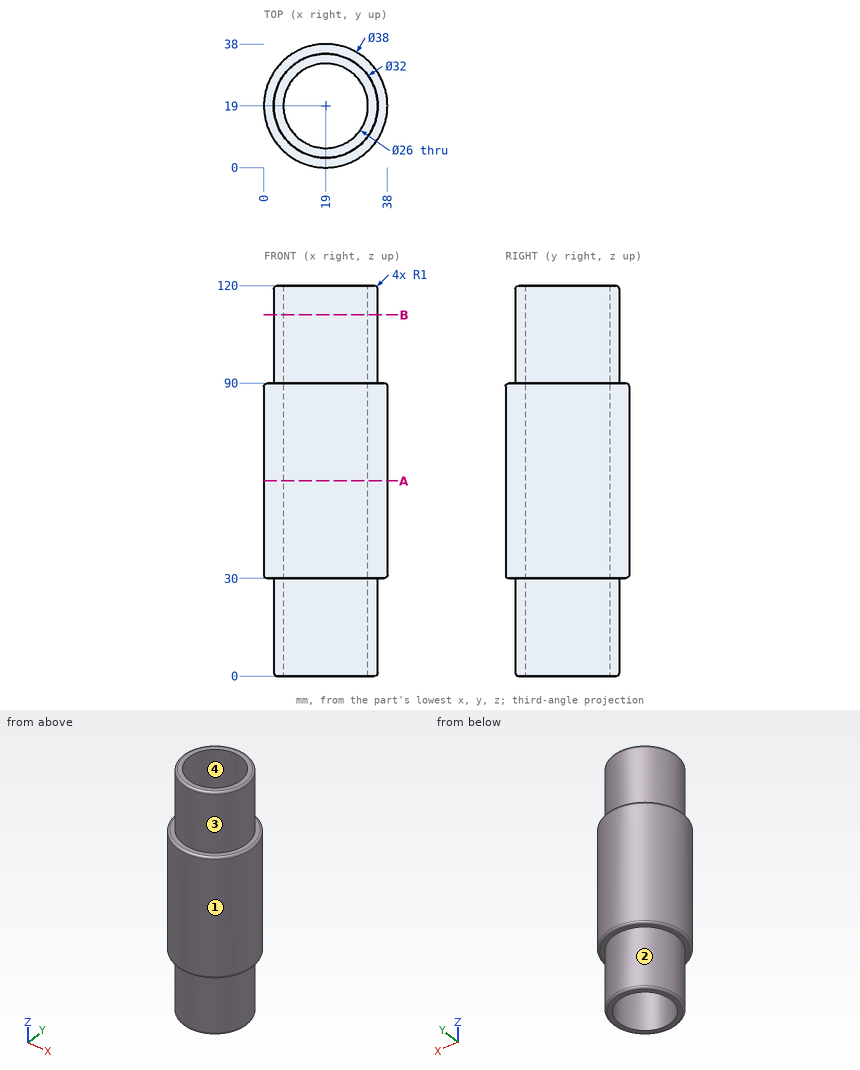
Can you work these out from the drawing? Everything is in mm from the part's minimum corner. A direction names the side the tool comes from. Round coordinates to 2 decimals unless told otherwise and drop trailing zeros. Loops run counter-clockwise (first coordinate to the right, second up) from the corner with the lowest first, then second, coordinate; pieces in that order, holes last. Notation, with made-up numbers: (78.25, 67) - (125.25, 67) arc R15 ccw to (125.25, 79) - close; hole circle Ø4 at (44.5, 52). An arc over 180 degrees is marked (long way). One line per question, with ' | ' between items. Start each with the question number.
Q1. Will these pins go through, and if not, where does the flat tip stop? pin 1 (4 mm diameter, centred on x = 20.5, z = 88.5, fed in from -Y); pin 2 (8 mm diameter, centred on x = 9, z = 54.5, fed in from -Y); pin 3 (8 mm diameter, centred on y = 29, z = 71, fed in from -X).
Q2. I want a section at B-B (z = 111). Write out the boundary of the cut face in (x, y).
Q3. We'd pull the mould along Y, two halves only. Please class the marked faces 3 and 4: +Y half, -Y half, draft (parallel to the pull), parting line (faces both ways), or undercut.
Q4. I want a section at A-A (z = 60). Write out the boundary of the cut face in (x, y).
Q5. Please list where these lines run through material, in increasing order: line 1 (Y direction, x = 19, z = 92.5); line 2 (Y direction, x = 19, z = 74.5); line 3 (X direction, y = 7, z = 72.5). Write a range as [from, to].
Q6. For the marked faces 1 and 2, which set-ups out of +Z, -Z, +X, -X, +Y, -Y let a thin tool reach every point of the face, with its end or its side?
Response values:
1) pin 1: stops at y = 0 | pin 2: stops at y = 0.97 | pin 3: stops at x = 0.97
2) outline: circle Ø32 at (19, 19); hole circle Ø26 at (19, 19)
3) face 3: parting line | face 4: undercut
4) outline: circle Ø38 at (19, 19); hole circle Ø26 at (19, 19)
5) line 1: y = [3, 6], [32, 35] | line 2: y = [0, 6], [32, 38] | line 3: x = [4.27, 14], [24, 33.73]
6) face 1: +Z, -Z | face 2: -Z
